```python
from build123d import *

# Parameters (mm, degrees)
SKETCH2_W           = 19
SKETCH2_H           = 19
BOSS_EXTRUDE1_DEPTH = 6
SKETCH3_R           = 4.5
BOSS_EXTRUDE2_DEPTH = 76


with BuildPart() as part:
    # Sketch2 → Boss-Extrude1 (new body)
    with BuildSketch(Plane(origin=(0, 0, 0), x_dir=(0, 0, -1), z_dir=(1, 0, 0))):
        with Locations((9.5, 9.5)):
            Rectangle(SKETCH2_W, SKETCH2_H)
    extrude(amount=BOSS_EXTRUDE1_DEPTH)

    # Sketch3 → Boss-Extrude2 (add)
    with BuildSketch(Plane.ZY):
        with Locations((-9.5, 9.5)):
            Circle(SKETCH3_R)
    extrude(amount=BOSS_EXTRUDE2_DEPTH)


solid = part.part
```
Design review of the part built by this model. Coordinates are the model's own, in mm. A direction names the side the tool comes from. Coordinates: 2 decimals unless noted, no trailing zeros. Write each loop counter-clockwise with the first axis right and the second up, starting at its lowest first coordinate (ties: lowest second). Pieces come first, ordered by that corner, then holes. Notation, with made-up numbers: M 79.5,21 L 136.5,21 A21 cw 136.5,41 Z; hole C 15,57.25 d3. An arc over 180 degrees is marked long. Answer as a JSON object with one key per item and string values.
Item 1: Machinability: for faces 1 (the cylindrical face through (-37.468, 10.852, -5.208)), 2 (the flat face through (3, 9, 0)), which of the approach directions +Z, -Z, +X, -X, +Y, -Y give a long, thin tool a straight path to every point of the face, cutting with its end or side? Answer none if there is none.
Outcome:
{"face 1": "-X", "face 2": "+Z, +X, -X, +Y, -Y"}
Item 2: Add section D-D, the plane y = 16.25. Give the boundary of the cut face in (x, z), and give its area (3 significant figures).
Outcome:
{"outline": "M 0,-19 L 6,-19 L 6,0 L 0,0 Z", "area": "114 mm²"}
Item 3: Insertion check: pin 1 Ø5 at (x, y) = (-14, 10.5) entering from -Z; pin 2 Ø6 at (y, z) = (13, -14) entering from -X; pin 3 Ø10 at (x, z) = (-5.5, -8.5) entering from +Y; pin 4 Ø4 at (x, y) = (-16.5, 15.5) entering from +Z. Each pin has a flat end and moves straight along its axis. Give the tip position at first contact, or say it passes through.
Outcome:
{"pin 1": "z = -14", "pin 2": "x = -76", "pin 3": "y = 14", "pin 4": "z = -7.44"}
Item 4: Add section C-C, the plane x = -65. Give the boundary of the cut face in (y, z), and give its area (3 significant figures).
Outcome:
{"outline": "C 9.5,-9.5 d9", "area": "63.6 mm²"}
Item 5: Wall thickness on probe 1 along X at (y, z) = (12.5, -2); probe 2 along Z at (x, y) = (-34, 9.25); probe 3 along Z at (x, y) = (-16, 8.25): over which ranges is each line inside the solid? List them lowest first.
Outcome:
{"probe 1": "0 to 6", "probe 2": "-13.99 to -5.01", "probe 3": "-13.82 to -5.18"}
Item 6: Add section B-B, the plane y = 9.5. Give the boundary of the cut face in (x, z), and give its area (3 significant figures).
Outcome:
{"outline": "M -76,-14 L 0,-14 L 0,-19 L 6,-19 L 6,0 L 0,0 L 0,-5 L -76,-5 Z", "area": "798 mm²"}
Item 7: Add section A-A, the plane z = -9.5. Give the boundary of the cut face in (x, y).
Outcome:
{"outline": "M -76,5 L 0,5 L 0,0 L 6,0 L 6,19 L 0,19 L 0,14 L -76,14 Z"}
